For this review, take the finished solid that the model builds, in its own axes (mm). A direction names the side the tool comes from. Give positions to 0.01 mm unless a question says otherwise; leave off trailing zeros. Write each loop counter-clockwise with the first axis right and the second up, starting at its lowest first coordinate (ties: lowest second). Pieces come first, ordered by that corner, then holes. Notation, with made-up numbers: M 48,-25.75 L 94,-25.75 A21 ccw 94,10.25 Z; hole C 77,58 d4. An arc over 180 degrees is marked long. One line per item, written item: value. Start each with the question number.
Item 1: To check wall thickness, follow probe 1 along Z at (x, y) = (26.54, 3.9); probe 2 along Z at (x, y) = (16.54, 4.05); probe 3 along Y at (x, z) = (2.54, -42.55). State the ranges of each line that lie inside material, in increasing order.
Item 2: Clearance check with flat-ended pins moving along their axes: pin 1 Ø4 at (x, y) = (30, -13.5) entering from +Z; pin 2 Ø1.5 at (x, y) = (1.5, -32.5) entering from +Z; pin 3 Ø1.7 at (x, y) = (30.54, -31.75) entering from -Z; pin 4 Ø4 at (y, z) = (3, -11.5) entering from -X. State where each tip first meets the part, or that it passes through.
Item 3: Tool access review of faces 4 (the face through (4.963, -3.047, -37.916)), 5 (the face through (32, -32, -35.34)), 6 (the face through (16, -35.56, -43)), 7 (the face through (30.54, 3, -18)): name each direction out of +Z, -Z, +X, -X, +Y, -Y from which nothing blocks a thin tool from reaching the whole face with its end or side.
Item 4: Consider section B-B, the plane y = -16.5. Write out the cut boundary in (x, z).
Item 5: Mouldability with a two-part tool opening along Y and no side actions: class faces 1 (the face through (2.21, -29.23, -37.92)), 2 (the face through (16, 5.08, -23)), 3 (the face through (33.08, -17, -43)) as released by +Y, released by -Y, zero draft, split by the parting line, or undercut.
Item 6: Consider section C-C, the plane x = 16.54. Write out the cut boundary in (y, z).
Item 7: Consider section D-D, the plane x = 23. Write out the cut boundary in (y, z), and give its area (3 significant figures).
Item 8: Consider section A-A, the plane z = -39. Give the number of separate pieces and of enclosed holes in the cut face, and give its area (3 significant figures).
```python
from build123d import *

# Parameters (mm, degrees)
SKETCH1_W               = 33.08
SKETCH1_H               = 45.5
BOSS_EXTRUDE1_DEPTH     = 5.08
SKETCH2_R               = 1.7
CUT_EXTRUDE1_DEPTH      = 6.08
SKETCH3_W               = 33.08
SKETCH3_H               = 5.08
BOSS_EXTRUDE2_DEPTH     = 40.64
SKETCH4_R               = 1.0795
SKETCH4_W               = 22.86
SKETCH4_H               = 35.56
CUT_EXTRUDE2_DEPTH      = 41.42
CUT_EXTRUDE2_DEPTH_BACK = 6.08
SKETCH5_R               = 2.54
SKETCH5_R_2             = 1.0795
BOSS_EXTRUDE3_DEPTH     = 5.08
SKETCH6_W               = 2.54
SKETCH6_H               = 35.34
CUT_EXTRUDE3_DEPTH      = 6.08


with BuildPart() as part:
    # Sketch1 → Boss-Extrude1 (new body)
    with BuildSketch(Plane(origin=(0, 0, 0), x_dir=(1, 0, 0), z_dir=(0, 1, 0))):
        with Locations((16.54, 22.75)):
            Rectangle(SKETCH1_W, SKETCH1_H)
    extrude(amount=BOSS_EXTRUDE1_DEPTH)

    # Sketch2 → Cut-Extrude1 (cut, through all)
    with BuildSketch(Plane.XZ):
        with Locations((6.54, -28.7)):
            Circle(SKETCH2_R)
        with Locations((26.54, -28.7)):
            Circle(SKETCH2_R)
        with Locations((16.54, -5)):
            Circle(SKETCH2_R)
    extrude(amount=-CUT_EXTRUDE1_DEPTH, mode=Mode.SUBTRACT)

    # Sketch3 → Boss-Extrude2 (add)
    with BuildSketch(Plane.XZ):
        with Locations((16.54, -42.96)):
            Rectangle(SKETCH3_W, SKETCH3_H)
    extrude(amount=BOSS_EXTRUDE2_DEPTH)

    # Sketch4 → Cut-Extrude2 (cut, two sides)
    with BuildSketch(Plane.XY.offset(-40.42)) as cut_extrude2_sk:
        with Locations((30.54, -31.75)):
            Circle(SKETCH4_R)
        with Locations((2.54, -31.75)):
            Circle(SKETCH4_R)
        with Locations((30.54, -3.81)):
            Circle(SKETCH4_R)
        with Locations((2.54, -3.81)):
            Circle(SKETCH4_R)
        with Locations((16.57, -17.78)):
            Rectangle(SKETCH4_W, SKETCH4_H)
    extrude(amount=CUT_EXTRUDE2_DEPTH, mode=Mode.SUBTRACT)
    extrude(cut_extrude2_sk.sketch, amount=-CUT_EXTRUDE2_DEPTH_BACK, mode=Mode.SUBTRACT)

    # Sketch5 → Boss-Extrude3 (add)
    with BuildSketch(Plane.XY.offset(-40.42)):
        with Locations((30.54, -31.75)):
            Circle(SKETCH5_R)
        with Locations((30.54, -31.75)):
            Circle(SKETCH5_R_2, mode=Mode.SUBTRACT)
        with Locations((30.54, -3.81)):
            Circle(SKETCH5_R)
        with Locations((30.54, -3.81)):
            Circle(SKETCH5_R_2, mode=Mode.SUBTRACT)
        with Locations((2.54, -3.81)):
            Circle(SKETCH5_R)
        with Locations((2.54, -3.81)):
            Circle(SKETCH5_R_2, mode=Mode.SUBTRACT)
        with Locations((2.54, -31.75)):
            Circle(SKETCH5_R)
        with Locations((2.54, -31.75)):
            Circle(SKETCH5_R_2, mode=Mode.SUBTRACT)
    extrude(amount=BOSS_EXTRUDE3_DEPTH)

    # Sketch6 → Cut-Extrude3 (cut, through all)
    with BuildSketch(Plane.XZ):
        with Locations((1.27, -17.67)):
            Rectangle(SKETCH6_W, SKETCH6_H)
        with Locations((31.81, -17.67)):
            Rectangle(SKETCH6_W, SKETCH6_H)
    extrude(amount=-CUT_EXTRUDE3_DEPTH, mode=Mode.SUBTRACT)


solid = part.part
```
Model answer:
1. probe 1: z = -45.5 to -30.4, -27 to 0
1. probe 2: z = -45.5 to -6.7, -3.3 to 0
1. probe 3: y = -40.64 to -32.83, -30.67 to -4.89, -2.73 to 5.08
2. pin 1: stops at z = -40.42
2. pin 2: stops at z = -35.34
2. pin 3: passes through
2. pin 4: stops at x = 2.54
3. face 4: +Z
3. face 5: +Z, +X, -X, -Y
3. face 6: +Z, -Z
3. face 7: +Z, +X, +Y, -Y
4. outline: M 0,-45.5 L 5.14,-45.5 L 5.14,-40.42 L 0,-40.42 Z; M 28,-45.5 L 33.08,-45.5 L 33.08,-40.42 L 28,-40.42 Z
5. face 1: undercut
5. face 2: released by +Y
5. face 3: zero draft
6. outline: M -40.64,-45.5 L -35.56,-45.5 L -35.56,-40.42 L -40.64,-40.42 Z; M 0,-45.5 L 5.08,-45.5 L 5.08,-6.7 L 0,-6.7 Z; M 0,-3.3 L 5.08,-3.3 L 5.08,0 L 0,0 Z
7. outline: M -40.64,-45.5 L -35.56,-45.5 L -35.56,-40.42 L -40.64,-40.42 Z; M 0,-45.5 L 5.08,-45.5 L 5.08,0 L 0,0 Z
7. area: 257 mm2
8. separate pieces: 5
8. enclosed holes: 4
8. area: 234 mm2
